Could you check a few things on this model? Use its own coordinates, in mm. Face numbers are marked on the shaded views. A direction names the side the tool comes from. Round coordinates to 2 decimals unless told otherwise and drop trailing zeros. Loops run counter-clockwise (first coordinate to the right, second up) from the corner with the lowest first, then second, coordinate; pieces in that order, holes last. Notation, with made-up numbers: (20.25, 84) -> (65.25, 84) arc R19 cw to (65.25, 117) -> close; hole circle Ø4 at (9, -2.5). An arc over 180 degrees is marked (long way). One line per item, written item: value.
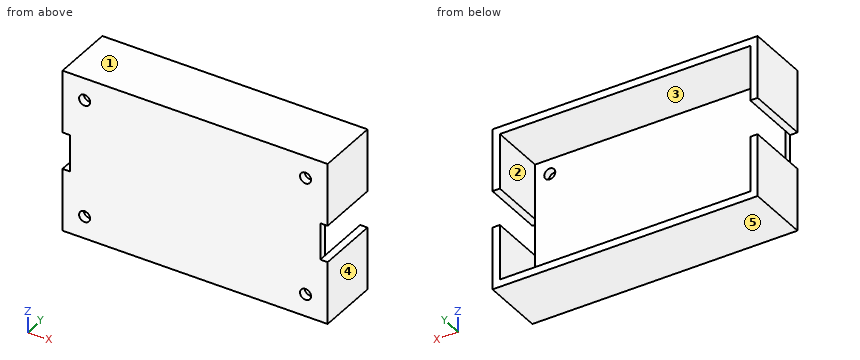
```python
from build123d import *

# Parameters (mm, degrees)
SKETCH_2_W          = 72
SKETCH_2_H          = 44
SKETCH_2_W_2        = 68
SKETCH_2_H_2        = 40
EXTRUDE_1_DEPTH     = 15
SKETCH_2_3_W        = 72
SKETCH_2_3_H        = 44
SKETCH_2_3_W_2      = 68
SKETCH_2_3_H_2      = 40
SKETCH_2_3_R        = 1.5
EXTRUDE_2_DEPTH     = 2
SKETCH_4_W          = 10
SKETCH_4_H          = 17
CUT_EXTRUDE_1_DEPTH = 2
SKETCH_5_W          = 10
SKETCH_5_H          = 17
CUT_EXTRUDE_2_DEPTH = 2


with BuildPart() as part:
    # Sketch 2 → Extrude 1 (new body)
    with BuildSketch(Plane(origin=(0, 0, 0), x_dir=(1, 0, 0), z_dir=(0, 1, 0))):
        with Locations((36, -22)):
            Rectangle(SKETCH_2_W, SKETCH_2_H)
        with Locations((36, -22)):
            Rectangle(SKETCH_2_W_2, SKETCH_2_H_2, mode=Mode.SUBTRACT)
    extrude(amount=EXTRUDE_1_DEPTH)

    # Sketch 2_3 → Extrude 2 (add)
    # profile 1 of 2: a face of its own
    with BuildSketch(Plane(origin=(0, 0, 0), x_dir=(1, 0, 0), z_dir=(0, 1, 0))):
        with Locations((36, -22)):
            Rectangle(SKETCH_2_3_W, SKETCH_2_3_H)
        with Locations((36, -22)):
            Rectangle(SKETCH_2_3_W_2, SKETCH_2_3_H_2, mode=Mode.SUBTRACT)
    # profile 2 of 2: a face of its own
    with BuildSketch(Plane(origin=(0, 0, 0), x_dir=(1, 0, 0), z_dir=(0, 1, 0))):
        with Locations((36, -22)):
            Rectangle(SKETCH_2_3_W_2, SKETCH_2_3_H_2)
        with Locations(Location((66, -6, 0), (0, 0, 270))):
            Circle(SKETCH_2_3_R, mode=Mode.SUBTRACT)
        with Locations(Location((6, -6, 0), (0, 0, 270))):
            Circle(SKETCH_2_3_R, mode=Mode.SUBTRACT)
        with Locations(Location((6, -38, 0), (0, 0, 270))):
            Circle(SKETCH_2_3_R, mode=Mode.SUBTRACT)
        with Locations(Location((66, -38, 0), (0, 0, 270))):
            Circle(SKETCH_2_3_R, mode=Mode.SUBTRACT)
    extrude(amount=-EXTRUDE_2_DEPTH)

    # Sketch 4 → Cut-Extrude 1 (cut)
    with BuildSketch(Plane.ZY):
        with Locations((22, 6.5)):
            Rectangle(SKETCH_4_W, SKETCH_4_H)
    extrude(amount=-CUT_EXTRUDE_1_DEPTH, mode=Mode.SUBTRACT)

    # Sketch 5 → Cut-Extrude 2 (cut)
    with BuildSketch(Plane(origin=(72, 0, 0), x_dir=(0, 0, -1), z_dir=(1, 0, 0))):
        with Locations((-22, 6.5)):
            Rectangle(SKETCH_5_W, SKETCH_5_H)
    extrude(amount=-CUT_EXTRUDE_2_DEPTH, mode=Mode.SUBTRACT)


solid = part.part
```
Item 1: If we section it at A-A on x = 66: List the corners of the cut face in (y, z) for me, plus the area to 3 significant figures.
Output:
outline: (-2, 0) -> (15, 0) -> (15, 2) -> (0, 2) -> (0, 4.5) -> (-2, 4.5) -> close; (-2, 7.5) -> (0, 7.5) -> (0, 36.5) -> (-2, 36.5) -> close; (-2, 39.5) -> (0, 39.5) -> (0, 42) -> (15, 42) -> (15, 44) -> (-2, 44) -> close
area: 136 mm²
Item 2: If we section it at D-D on z = 15: List the corners of the cut face in (x, y) for me.
Output:
outline: (0, -2) -> (72, -2) -> (72, 15) -> (70, 15) -> (70, 0) -> (2, 0) -> (2, 15) -> (0, 15) -> close
Item 3: If we section it at C-C on z = 38: List the corners of the cut face in (x, y) for me.
Output:
outline: (0, -2) -> (4.5, -2) -> (4.5, 0) -> (2, 0) -> (2, 15) -> (0, 15) -> close; (7.5, -2) -> (64.5, -2) -> (64.5, 0) -> (7.5, 0) -> close; (67.5, -2) -> (72, -2) -> (72, 15) -> (70, 15) -> (70, 0) -> (67.5, 0) -> close
Item 4: Will these pins go through, and if not, where does the flat tip stop? pin 1 Ø6 at (x, z) = (28, 36) entering from +Y; pin 2 Ø1.8 at (x, z) = (6, 6) entering from +Y; pin 3 Ø0.6 at (y, z) = (-1.5, 21.5) entering from +X; pin 4 Ø1 at (y, z) = (-0.5, 20) entering from -X.
Output:
pin 1: stops at y = 0
pin 2: passes through
pin 3: stops at x = 70
pin 4: stops at x = 2
Item 5: If we mould it in two halves opening along X, with no side actions, what happens to the marked faces 3, 4 and 5? For each: released by +X, released by -X, zero draft, split by the parting line, or undercut.
Output:
face 3: undercut
face 4: released by +X
face 5: zero draft
Item 6: For the marked faces 1 and 2, which set-ups out of +Z, -Z, +X, -X, +Y, -Y let a thin tool reach every point of the face, with its end or its side?
Output:
face 1: +Z, +X, -X, +Y, -Y
face 2: +Y
Item 7: I need wall thicknesses on line 1 (X direction, y = -1.1, z = 6); line 2 (Z direction, x = 66, y = -0.45); line 3 (X direction, y = 7.5, z = 40.5). Which ranges of each line are inside material? Lowest first, please. Write a range as from..to.
Output:
line 1: x = 0..4.5, 7.5..64.5, 67.5..72
line 2: z = 0..4.5, 7.5..36.5, 39.5..44
line 3: x = 0..2, 70..72
Item 8: If we section it at B-B on y = 9.25: List the corners of the cut face in (x, z) for me.
Output:
outline: (0, 0) -> (72, 0) -> (72, 17) -> (70, 17) -> (70, 2) -> (2, 2) -> (2, 17) -> (0, 17) -> close; (0, 27) -> (2, 27) -> (2, 42) -> (70, 42) -> (70, 27) -> (72, 27) -> (72, 44) -> (0, 44) -> close
